Geometry: see drawing. Coordinates: mm, zero at the bounding-box minimum. A direction names the side the tool comes from. Coordinates: 2 decimals unless noted, no trailing zeros. Write each loop counter-clockwise with the first axis right and the second up, starting at its lowest first coordinate (ties: lowest second). Pieces come first, ordered by that corner, then holes.
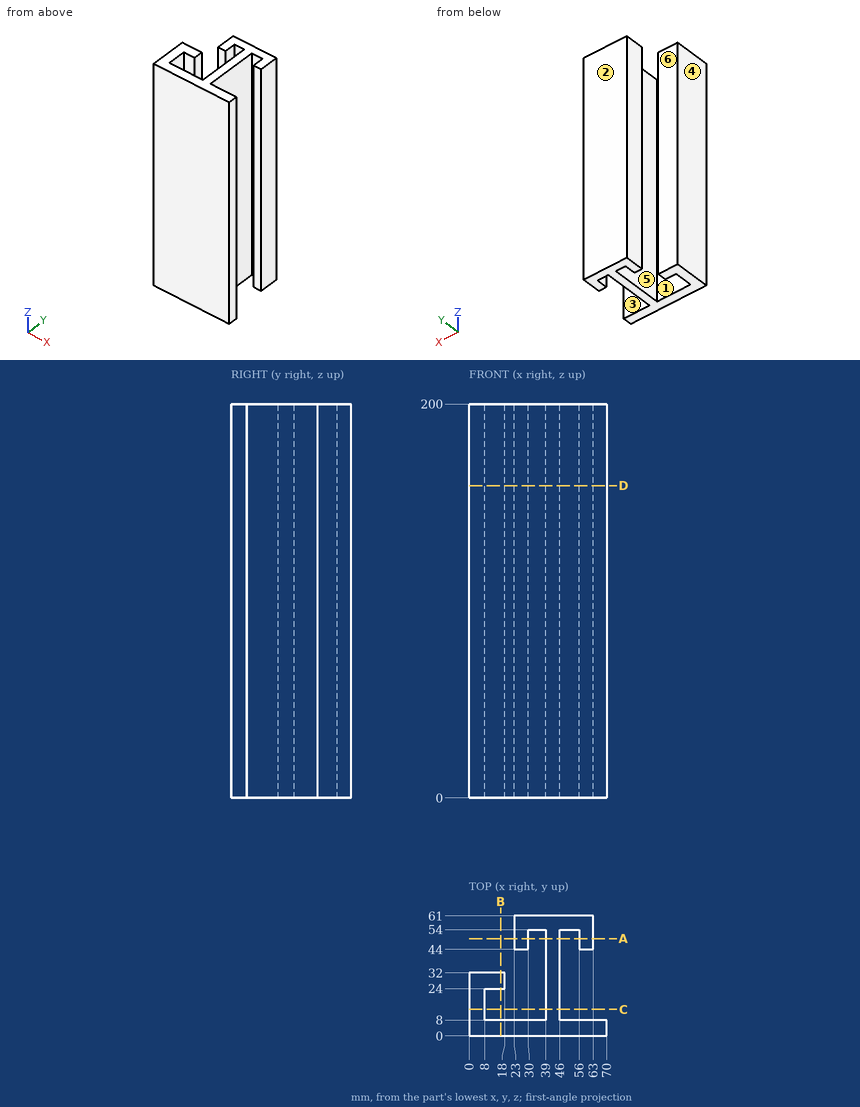
Item 1: Section C-C, the plane y = 13.5. Output: boundary loops of the cut face in (x, z), plus the area to 3 significant figures.
Derived:
outline: (0, 0) - (8, 0) - (8, 200) - (0, 200) - close; (39, 0) - (46, 0) - (46, 200) - (39, 200) - close
area: 3,000 mm2
Item 2: Section D-D, the plane z = 158.5. Output: boundary loops of the cut face in (x, y), plus the area to 3 significant figures.
Derived:
outline: (0, 0) - (70, 0) - (70, 8) - (46, 8) - (46, 54) - (56, 54) - (56, 44) - (63, 44) - (63, 61) - (23, 61) - (23, 44) - (30, 44) - (30, 54) - (39, 54) - (39, 8) - (8, 8) - (8, 24) - (18, 24) - (18, 32) - (0, 32) - close
area: 1,570 mm2
Item 3: Material intervals for probe 1 along X at (y, z) = (49.5, 63); probe 2 along X at (y, z) = (27.5, 160); probe 3 along X at (y, z) = (23, 106), sorted ascending.
Derived:
probe 1: x = 23 to 30, 39 to 46, 56 to 63
probe 2: x = 0 to 18, 39 to 46
probe 3: x = 0 to 8, 39 to 46
Item 4: Pin query (flat end, axial travel): pin 1 (5 mm diameter, centred on y = 54.5, z = 94.5, fed in from +X); pin 2 (3 mm diameter, centred on y = 50, z = 117.5, fed in from -X); pin 3 (9 mm diameter, centred on x = 12, z = 132.5, fed in from +Y). Return the tip coordinate at first contact, or that it passes through.
Derived:
pin 1: stops at x = 63
pin 2: stops at x = 23
pin 3: stops at y = 32
Item 5: Section A-A, the plane y = 49.5. Output: boundary loops of the cut face in (x, z).
Derived:
outline: (23, 0) - (30, 0) - (30, 200) - (23, 200) - close; (39, 0) - (46, 0) - (46, 200) - (39, 200) - close; (56, 0) - (63, 0) - (63, 200) - (56, 200) - close
Item 6: Set-up query: the marked faces 1, 2 and 3. Return all of +Z, -Z, +X, -X, +Y, -Y with unobstructed straight access to the full face (end or side cutting, diameter ignored); none if empty.
Derived:
face 1: +Z, -Z
face 2: +Z, -Z, +X, -X, +Y
face 3: +Z, -Z, +X
Item 7: Pull-direction query (X, two-part tool) for the marked faces 4, 5 and 6; classes: released by +X, released by -X, zero draft, split by the parting line, or undercut.
Derived:
face 4: released by -X
face 5: undercut
face 6: zero draft
Item 8: Section B-B, the plane x = 16. Output: boundary loops of the cut face in (y, z).
Derived:
outline: (0, 0) - (8, 0) - (8, 200) - (0, 200) - close; (24, 0) - (32, 0) - (32, 200) - (24, 200) - close
